```python
from build123d import *

# Parameters (mm, degrees)
SKETCH1_W           = 24.499964053
SKETCH1_H           = 13.5
BOSS_EXTRUDE1_DEPTH = 1.9
CHAMFER2_SIZE       = 1.5
SKETCH3_W           = 4.970239213
SKETCH3_H           = 5
SKETCH3_W_2         = 5.304118475
SKETCH3_H_2         = 3.940048439
SKETCH3_H_3         = 4.081751912
BOSS_EXTRUDE4_DEPTH = 1.5


with BuildPart() as part:
    # Sketch1 → Boss-Extrude1 (new body)
    with BuildSketch(Plane.XY):
        Polygon((5.471235903, 20.676320824), (40.471199956, 20.726483376), (40.471199956, 2.164736428), (40.316871719, -3.053294073), (39.006131301, -12.842886574), (38.115574665, -19.494231445), (37.577206439, -19.494231445), (8.577206439, -19.494231445), (7.251992344, -12.950986849), (5.926778248, -3.053294073), (5.471235903, 2.164736428), align=None)
        with Locations((22.971217929, -0.023516624)):
            Rectangle(SKETCH1_W, SKETCH1_H, mode=Mode.SUBTRACT)
    extrude(amount=BOSS_EXTRUDE1_DEPTH)

    # Chamfer2
    chamfer2_edges = [part.edges().sort_by_distance(p)[0] for p in [
        (22.971217929, 6.726483376, 1.9),
        (22.971217929, -6.773516624, 1.9),
    ]]
    chamfer(chamfer2_edges, length=CHAMFER2_SIZE)

    # Sketch3 → Boss-Extrude4 (add)
    with BuildSketch(Plane(origin=(0, 0, 0), x_dir=(-1, 0, 0), z_dir=(0, 0, -1))):
        with Locations((-32.736080349, -9.273516624)):
            Rectangle(SKETCH3_W, SKETCH3_H)
        with Locations((-13.343741273, -9.273516624)):
            Rectangle(SKETCH3_W_2, SKETCH3_H)
        with Locations((-32.736080349, 12.652087829)):
            Rectangle(SKETCH3_W, SKETCH3_H_2)
        with Locations((-13.343741273, 12.581236092)):
            Rectangle(SKETCH3_W_2, SKETCH3_H_3)
    extrude(amount=BOSS_EXTRUDE4_DEPTH)


solid = part.part
```
Work out the finished part from the listing and answer in its coordinate system (mm). A direction names the side the tool comes from. Coordinates: 2 decimals unless noted, no trailing zeros. Write each loop counter-clockwise with the first axis right and the second up, starting at its lowest first coordinate (ties: lowest second). Pieces come first, ordered by that corner, then holes.
Q1. A cutting plane is placed at A-A, the plane y = 3. Give the vertices of the cut face in (x, z), then the cut area to 4 significant figures.
Q2. A cutting plane is placed at D-D, the plane z = 1.45. Give the vertices of the cut face in (x, y), then the cut area to 3 significant figures.
Q3. A cutting plane is placed at C-C, the plane x = 18. Give the vertices of the cut face in (y, z).
Q4. A cutting plane is placed at B-B, the plane z = -0.6. Give the vertices of the cut face in (x, y), then the cut area to 3 significant figures.
Q5. Find the intervals of material crossed by line 1 (Z direction, x = 29, y = 13); line 2 (Y direction, x = 22, z = 1.1); line 3 (Y direction, x = 13, z = 1.5), in increasing order.
Q6. Each of these flat-tipped pins is pushed along its axis until it touches: pin 1 Ø0.8 at (x, z) = (32.5, -1) entering from -Y; pin 2 Ø1.6 at (y, z) = (13, -1) entering from +X; pin 3 Ø1.6 at (y, z) = (-9, -1) entering from -X; pin 4 Ø1 at (x, z) = (24, -1) entering from -Y. Where does it stop, or does it pass through?
Q7. Determine the mould class of faces 4 (the face through (40.471, 12, 1)), 5 (the face through (15.996, 13, -1)), 6 (the face through (10.721, 0, 1)), 7 (the face through (7.924, -16.268, 0.937)) for opening direction X: released by +X, released by -X, zero draft, split by the parting line, or undercut.
Q8. Which of the six approach directions +Z, -Z, +X, -X, +Y, -Y give full straight-line access (tool end or side, diameter ignored) to faces 1 (the face through (13, 14.622, -1)), 2 (the face through (35.221, 13, -1)), 3 (the face through (33, 10.682, -1))?
Findings below:
1. outline: (5.47, 0) - (10.72, 0) - (10.72, 1.9) - (5.47, 1.9) - close; (35.22, 0) - (40.47, 0) - (40.47, 1.9) - (35.22, 1.9) - close
1. area: 19.95 mm2
2. outline: (5.47, 2.16) - (5.93, -3.05) - (7.25, -12.95) - (8.58, -19.49) - (38.12, -19.49) - (40.32, -3.05) - (40.47, 2.16) - (40.47, 20.73) - (5.47, 20.68) - close; hole (10.72, -7.82) - (35.22, -7.82) - (35.22, 7.78) - (10.72, 7.78) - close
2. area: 975 mm2
3. outline: (-19.49, 0) - (-6.77, 0) - (-6.77, 0.4) - (-8.27, 1.9) - (-19.49, 1.9) - close; (6.73, 0) - (20.69, 0) - (20.69, 1.9) - (8.23, 1.9) - (6.73, 0.4) - close
4. outline: (10.69, -11.77) - (16, -11.77) - (16, -6.77) - (10.69, -6.77) - close; (10.69, 10.54) - (16, 10.54) - (16, 14.62) - (10.69, 14.62) - close; (30.25, -11.77) - (35.22, -11.77) - (35.22, -6.77) - (30.25, -6.77) - close; (30.25, 10.68) - (35.22, 10.68) - (35.22, 14.62) - (30.25, 14.62) - close
4. area: 92.6 mm2
5. line 1: z = 0 to 1.9
5. line 2: y = -19.49 to -7.47, 7.43 to 20.7
5. line 3: y = -19.49 to -7.87, 7.83 to 20.69
6. pin 1: stops at y = -11.77
6. pin 2: stops at x = 35.22
6. pin 3: stops at x = 10.69
6. pin 4: passes through
7. face 4: released by +X
7. face 5: undercut
7. face 6: undercut
7. face 7: released by -X
8. face 1: -Z, +X, -X, +Y
8. face 2: -Z, +X, +Y, -Y
8. face 3: -Z, +X
